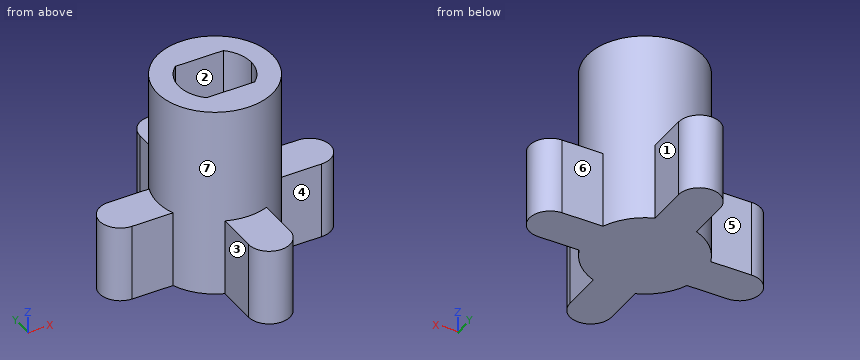
from build123d import *

# Parameters (mm, degrees)
F0_R          = 4.7625
F1_DEPTH      = 9.525
F1_DEPTH_BACK = 6.35
F4_DEPTH      = 9.526
F6_DEPTH      = 6.35
F7_COUNT      = 4


with BuildPart() as f1:
    # F0 (on Top) → F1 (new body, two sides)
    with BuildSketch(Plane.XY) as f1_sk:
        Circle(F0_R)
    extrude(amount=F1_DEPTH)
    extrude(f1_sk.sketch, amount=-F1_DEPTH_BACK)

    # F2 (on Top) → F4 (cut, through all)
    with BuildSketch(Plane.XY):
        with BuildLine():
            ThreePointArc((1.9843134833, -2.25), (2.7343134833, -1.2343134833), (3, 0))
            ThreePointArc((3, 0), (2.7343134833, 1.2343134833), (1.9843134833, 2.25))
            Line((1.9843134833, 2.25), (-1.9843134833, 2.25))
            ThreePointArc((-1.9843134833, 2.25), (-3, 0), (-1.9843134833, -2.25))
            Line((-1.9843134833, -2.25), (1.9843134833, -2.25))
        make_face()
    extrude(amount=F4_DEPTH, mode=Mode.SUBTRACT)



with BuildPart() as f6:
    # F5 (on Top) → F6 (new body, through all)
    with BuildSketch(Plane.XY):
        with BuildLine():
            Line((0, 1.7145), (-7.8105, 1.7145))
            ThreePointArc((-7.8105, 1.7145), (-9.525, 0), (-7.8105, -1.7145))
            Line((-7.8105, -1.7145), (0, -1.7145))
            Line((0, -1.7145), (0, 1.7145))
        make_face()
    extrude(amount=-F6_DEPTH)


with BuildPart() as f1_1:
    add(f1.part)

    add(f6.part)  # F7 merges F6
    # F7: F6 ×4 about axis
    f7_axis = Axis((0, 0, 0), (0, 0, -1))
    for i in range(1, F7_COUNT):
        add(f6.part.rotate(f7_axis, i * 360 / F7_COUNT))


solid = f1_1.part
The listing builds one solid part. Answer for the finished solid, in the listing's coordinates (mm). Face numbers are marked on the shaded views. A direction names the side the tool comes from. Give positions to 0.01 mm unless a question says otherwise; leave off trailing zeros. Write each loop counter-clockwise with the first axis right and the second up, starting at its lowest first coordinate (ties: lowest second). Pieces come first, ordered by that corner, then holes. Notation, with made-up numbers: (7.25, -20) - (61.25, -20) arc R30 cw to (61.25, 17) - close; hole circle Ø7 at (-8.75, 59.25). An arc over 180 degrees is marked (long way). One line per question, with ' | ' between items. Start each with the question number.
1. Determine the mould class of the marked faces 1, 2, 3 and 4 for opening direction X: +X half, -X half, draft (parallel to the pull), parting line (faces both ways), or undercut.
2. For the marked faces 5, 6 and 7, determine the directions among +Z, -Z, +X, -X, +Y, -Y from which every point of the face is accessible in a straight line to the end or side of a thin tool.
3. Straight lines are drawn through the part: line 1 (Z direction, x = -8.25, y = -1.25); line 2 (X direction, y = -0.25, z = 2); line 3 (X direction, y = -1.5, z = 2.75). For each, find the intervals that lie inside material, in ascending order.
4. Section B-B, the plane z = -4 is taken. Determine the outline of the cut face in (x, y) (1 decimal).
5. Given P1, Ø2, axis at x = -1.5, y = -1, coming from the +Z side; P2, Ø3.5, axis at x = 6.5, z = -4.5, coming from the -Y side; P3, Ø1.2, axis at x = -0.5, z = 3, coming from the -Y side, each flat-ended and moving along its own axis, determine where each tip first touches the part or whether it passes through.
6. Section D-D, the plane y = -6.25 is taken. Determine the outline of the cut face in (x, z), then the cut area to 3 significant figures.
Result:
1) face 1: +X half | face 2: undercut | face 3: -X half | face 4: draft
2) face 5: +Z, -Z, -X, +Y | face 6: +Z, -Z, +X, +Y | face 7: +Z
3) line 1: z = -6.35 to 0 | line 2: x = -4.76 to -2.99, 2.99 to 4.76 | line 3: x = -4.52 to -2.6, 2.6 to 4.52
4) outline: (-7.8, -1.7) - (-4.4, -1.7) arc R4.8 ccw to (-1.7, -4.4) - (-1.7, -7.8) arc R1.7 ccw to (1.7, -7.8) - (1.7, -4.4) arc R4.8 ccw to (4.4, -1.7) - (7.8, -1.7) arc R1.7 ccw to (7.8, 1.7) - (4.4, 1.7) arc R4.8 ccw to (1.7, 4.4) - (1.7, 7.8) arc R1.7 ccw to (-1.7, 7.8) - (-1.7, 4.4) arc R4.8 ccw to (-4.4, 1.7) - (-7.8, 1.7) arc R1.7 ccw to start
5) P1: stops at z = 0 | P2: stops at y = -1.71 | P3: stops at y = -4.76
6) outline: (-1.71, -6.35) - (1.71, -6.35) - (1.71, 0) - (-1.71, 0) - close | area: 21.8 mm2
